Source: three-view drawing plus pictorial views. Frame: mm from the lowest corner of the part. Give positions to 0.01 mm unless a question says otherwise; leave off trailing zeros. Loops run counter-clockwise (first coordinate to the right, second up) from the corner with the lowest first, then second, coordinate; pieces in that order, holes last.
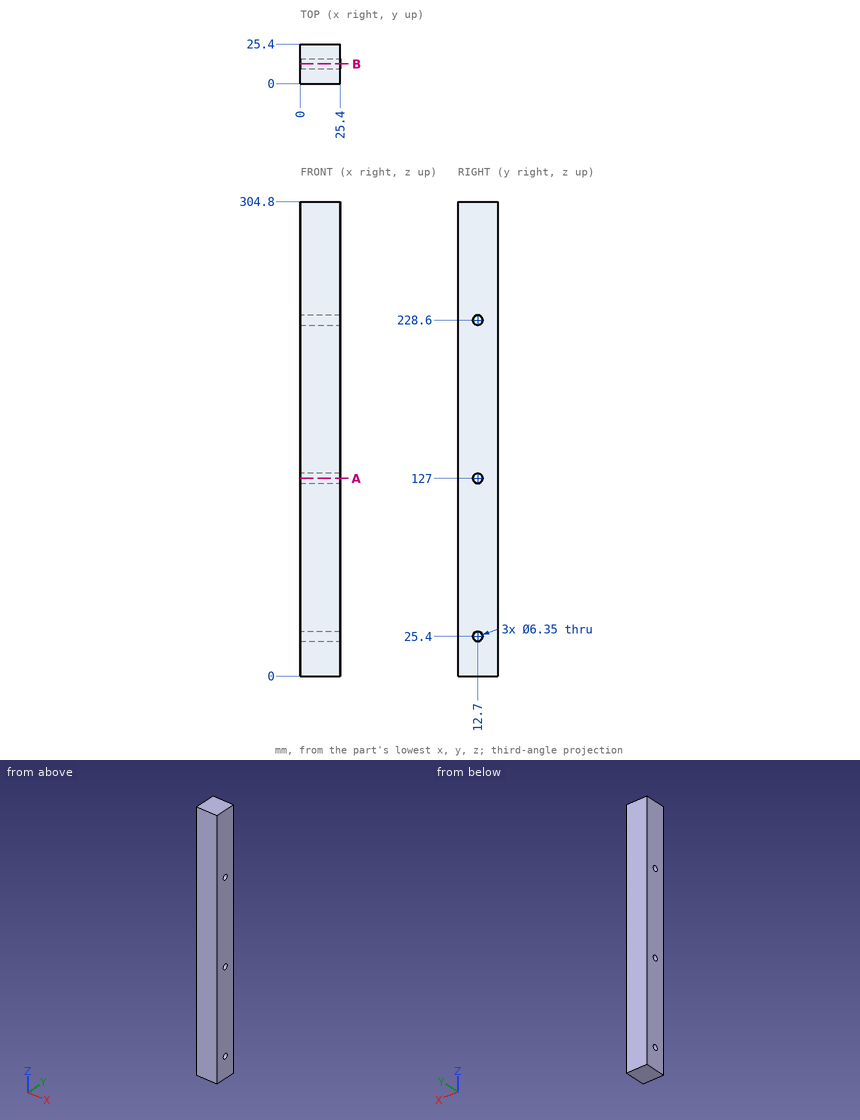
1) Cut plane B-B (y = 12.7). Return loops of the section in (x, z) (3 decimals), and give its area (3 significant figures).
Checks:
outline: (0, 0) - (25.4, 0) - (25.4, 22.225) - (0, 22.225) - close; (0, 28.575) - (25.4, 28.575) - (25.4, 123.825) - (0, 123.825) - close; (0, 130.175) - (25.4, 130.175) - (25.4, 225.425) - (0, 225.425) - close; (0, 231.775) - (25.4, 231.775) - (25.4, 304.8) - (0, 304.8) - close
area: 7,260 mm2
2) Cut plane A-A (z = 127). Return loops of the section in (x, y) (3 decimals).
Checks:
outline: (0, 0) - (25.4, 0) - (25.4, 9.525) - (0, 9.525) - close; (0, 15.875) - (25.4, 15.875) - (25.4, 25.4) - (0, 25.4) - close
3) Ray query, probe 1 along Z at (x, y) = (15, 12.7) (3 decimals); probe 2 along Y at (x, z) = (15.25, 25.4) (3 decimals); probe 3 along Z at (x, y) = (21, 10.25). Return the intervals inside material, ascending.
Checks:
probe 1: z = 0 to 22.225, 28.575 to 123.825, 130.175 to 225.425, 231.775 to 304.8
probe 2: y = 0 to 9.525, 15.875 to 25.4
probe 3: z = 0 to 23.38, 27.42 to 124.98, 129.02 to 226.58, 230.62 to 304.8
4) Contact query for a flat-ended pin moving along its axis: P1, Ø4, axis at y = 19, z = 94, coming from the -X side. Output: stop coordinate, or through.
Checks:
P1: stops at x = 0
